Autodesk Inventor part; units mm, degrees
ref_plane "YZ Plane" through (0, 0, 0) normal (1, 0, 0) x (0, 1, 0)
ref_plane "XZ Plane" through (0, 0, 0) normal (0, 1, 0) x (-1, 0, 0)
ref_plane "XY Plane" through (0, 0, 0) normal (0, 0, 1) x (1, 0, 0)
sketch "Sketch1" plane through (0, 0, 0) normal (0, 0, 1) x (1, 0, 0)
  line L0 (0, 15.666) -> (0, -15.666)
  line L1 (-34.4366, 0) -> (128.2896, 0)
  line L2 (0, 0) -> (93.853, 0) construction
  line L3 (0, 8.89) -> (93.853, 8.89)
  line L4 (0, -8.89) -> (93.853, -8.89)
  arc A0 (0, 8.89) -> (0, -8.89) centre (0, 0) ccw
  arc A1 (93.853, -8.89) -> (93.853, 8.89) centre (93.853, 0) ccw
  line L5 (93.853, 11.19) -> (0, 11.19)
  arc A2 (0, 11.19) -> (0, -11.19) centre (0, 0) ccw
  line L6 (0, -11.19) -> (93.853, -11.19)
  arc A3 (93.853, -11.19) -> (93.853, 11.19) centre (93.853, 0) ccw
  dimension "d0" = 93.853
  dimension "d5" = 8.89
  dimension "d6" = 8.89
  dimension "d7" = 2.3
extrude "Extrusion1" add sketch "Sketch1" along normal blind 9.525 contours L5 A3 L1 A1 L3 L0 | L0 A0 L1 A2 | L1 A0 L0 A2 | A3 L6 L0 L4 A1 L1
properties part number "BBP MCMASTER 1679K116_BELT"
Verification items for the finished model (mm, model axes). A direction names the side the tool comes from. Coordinates: 2 decimals unless noted, no trailing zeros. Loops run counter-clockwise (first coordinate to the right, second up) from the corner with the lowest first, then second, coordinate; pieces in that order, holes last. Notation, with made-up numbers: (-10, 37.25) -> (25, 37.25) arc R26 ccw to (25, 74.25) -> close; hole circle Ø6 at (-34, 41). An arc over 180 degrees is marked (long way). Answer in a Markdown table with one row per item.
1) Access from +Z, -Z, +X, -X, +Y, -Y to the whole of each face (thin tool, end or side, straight path). Record for faces 1 (the face through (102.74, 0.2, 4.7)), 2 (the face through (48, 11.19, 5)).
The answers:
| item | result |
|---|---|
| face 1 | +Z, -Z |
| face 2 | +Z, -Z, +X, -X, +Y |
2) Scan lines: line 1 along Y through (x, z) = (6, 5); line 2 along X through (y, z) = (6.25, 2); line 3 along X through (y, z) = (-7.5, 3.25). Record each from-to range of solid material in increasing order. Write a range as from..to.
The answers:
| item | result |
|---|---|
| line 1 | y = -11.19..-8.89, 8.89..11.19 |
| line 2 | x = -9.28..-6.32, 100.18..103.13 |
| line 3 | x = -8.3..-4.77, 98.63..102.16 |
3) Section check C-C (z = 3.5). Record the cut outline in (x, y).
The answers:
| item | result |
|---|---|
| outline | (0, -11.19) -> (93.85, -11.19) arc R11.19 ccw to (93.85, 11.19) -> (0, 11.19) arc R11.19 ccw to start; hole (0, -8.89) -> (93.85, -8.89) arc R8.89 ccw to (93.85, 8.89) -> (0, 8.89) arc R8.89 ccw to start |
4) Section check A-A (y = 0). Record the cut outline in (x, z) (3 decimals).
The answers:
| item | result |
|---|---|
| outline | (-11.19, 0) -> (-8.89, 0) -> (-8.89, 9.525) -> (-11.19, 9.525) -> close; (102.743, 0) -> (105.043, 0) -> (105.043, 9.525) -> (102.743, 9.525) -> close |
5) Section check B-B (x = 90). Record the cut outline in (y, z) (3 decimals), and give its area (3 significant figures).
The answers:
| item | result |
|---|---|
| outline | (-11.19, 0) -> (-8.89, 0) -> (-8.89, 9.525) -> (-11.19, 9.525) -> close; (8.89, 0) -> (11.19, 0) -> (11.19, 9.525) -> (8.89, 9.525) -> close |
| area | 43.8 mm2 |
